```python
from build123d import *

# Parameters (mm, degrees)
SKETCH1_R           = 3.175
BOSS_EXTRUDE1_DEPTH = 20
SKETCH2_R           = 1.675
CUT_EXTRUDE1_DEPTH  = 12
SKETCH4_R           = 6.35
BOSS_EXTRUDE2_DEPTH = 2.54
SKETCH6_R           = 6.35
BOSS_EXTRUDE3_DEPTH = 3.35


with BuildPart() as part:
    # Sketch1 → Boss-Extrude1 (new body)
    with BuildSketch(Plane(origin=(0, 0, 0), x_dir=(1, 0, 0), z_dir=(0, 1, 0))):
        Circle(SKETCH1_R)
    extrude(amount=BOSS_EXTRUDE1_DEPTH)

    # Sketch2 → Cut-Extrude1 (cut)
    with BuildSketch(Plane.XZ):
        Circle(SKETCH2_R)
    extrude(amount=-CUT_EXTRUDE1_DEPTH, mode=Mode.SUBTRACT)

    # Sketch4 → Boss-Extrude2 (add)
    with BuildSketch(Plane(origin=(0, 20, 0), x_dir=(1, 0, 0), z_dir=(0, 1, 0))):
        Circle(SKETCH4_R)
    extrude(amount=BOSS_EXTRUDE2_DEPTH)

    # Sketch6 → Boss-Extrude3 (add)
    with BuildSketch(Plane(origin=(0, 22.54, 0), x_dir=(1, 0, 0), z_dir=(0, 1, 0))):
        Circle(SKETCH6_R)
    extrude(amount=-BOSS_EXTRUDE3_DEPTH)


solid = part.part
```
Geometry check sheet. Reference: the model listing, model coordinates, mm. A direction names the side the tool comes from. Round coordinates to 2 decimals unless told otherwise and drop trailing zeros. Order: outer loops, then holes, each group sorted by start corner. A loop starts at its lowest first (then second) coordinate and runs counter-clockwise, first axis right, second up. Notation, with made-up numbers: (38, 46.25) - (94, 46.25) arc R31 cw to (94, 70.25) - close; hole circle Ø7 at (-27, -38). An arc over 180 degrees is marked (long way). Use a Markdown table: item, result. Add a question column.
1) Thickness scan on line 1 along Z through (x, y) = (0, 4.25) (3 decimals); line 2 along Y through (x, z) = (-4.25, -2); line 3 along X through (y, z) = (11.25, -1). Record the ranges inside material, lowest first.
2) Set-up check for faces 4 (the cylindrical face through (-0.69, 9.46, 3.1)), 5 (the flat face through (1.4, 0, 1.4)): record each of +Z, -Z, +X, -X, +Y, -Y from which the full face is reachable in a straight line by a thin tool's end or side.
3) Section check D-D (y = 7). Record the cut outline in (x, z) (3 decimals), then the cut area to 3 significant figures.
4) Gauge pin test, flat ends, axial feed: P1, Ø1, axis at x = 0, z = 0, coming from the -Y side; P2, Ø3, axis at y = 19, z = 2.5, coming from the -X side; P3, Ø6, axis at x = 2.5, y = 9, coming from the -Z side (3 decimals); P4, Ø1, axis at y = 3.5, z = 4, coming from the -X side. Record the tip position at first contact, or that the pin passes through.
5) Section check C-C (y = 17.75). Record the cut outline in (x, z) (3 decimals), then the cut area to 3 significant figures.
6) Section check A-A (z = 0). Record the cut outline in (x, y) (3 decimals).
7) Section check B-B (x = 0). Record the cut outline in (y, z) (3 decimals).
8) Mould release check, pull along Z, two halves, no side actions. Record for faces 1 (the cylindrical face through (-1.38, 20.84, 6.2)), 2 (the flat face through (0, 22.54, 0)), 3 (the cylindrical face through (-1.673, 5.916, 0.074)): released by +Z, released by -Z, zero draft, split by the parting line, or undercut.
Established:
| question | item | result |
|---|---|---|
| 1 | line 1 | -3.175 to -1.675, 1.675 to 3.175 |
| 1 | line 2 | 19.19 to 22.54 |
| 1 | line 3 | -3.01 to -1.34, 1.34 to 3.01 |
| 2 | face 4 | -Y |
| 2 | face 5 | +Z, -Z, +X, -X, -Y |
| 3 | outline | circle Ø6.35 at (0, 0); hole circle Ø3.35 at (0, 0) |
| 3 | area | 22.9 mm2 |
| 4 | P1 | y = 12 |
| 4 | P2 | x = -6.27 |
| 4 | P3 | z = -3.175 |
| 4 | P4 | through |
| 5 | outline | circle Ø6.35 at (0, 0) |
| 5 | area | 31.7 mm2 |
| 6 | outline | (-6.35, 19.19) - (-3.175, 19.19) - (-3.175, 0) - (-1.675, 0) - (-1.675, 12) - (1.675, 12) - (1.675, 0) - (3.175, 0) - (3.175, 19.19) - (6.35, 19.19) - (6.35, 22.54) - (-6.35, 22.54) - close |
| 7 | outline | (0, -3.175) - (19.19, -3.175) - (19.19, -6.35) - (22.54, -6.35) - (22.54, 6.35) - (19.19, 6.35) - (19.19, 3.175) - (0, 3.175) - (0, 1.675) - (12, 1.675) - (12, -1.675) - (0, -1.675) - close |
| 8 | face 1 | split by the parting line |
| 8 | face 2 | zero draft |
| 8 | face 3 | undercut |
